Drawing for the job (mm, zero at the part's lowest x, y, z). A direction names the side the tool comes from. Give positions to 0.01 mm unless a question says otherwise; leave off trailing zeros. Write each loop counter-clockwise with the first axis right and the second up, starting at its lowest first coordinate (ties: lowest second). Pieces come first, ordered by that corner, then holes.
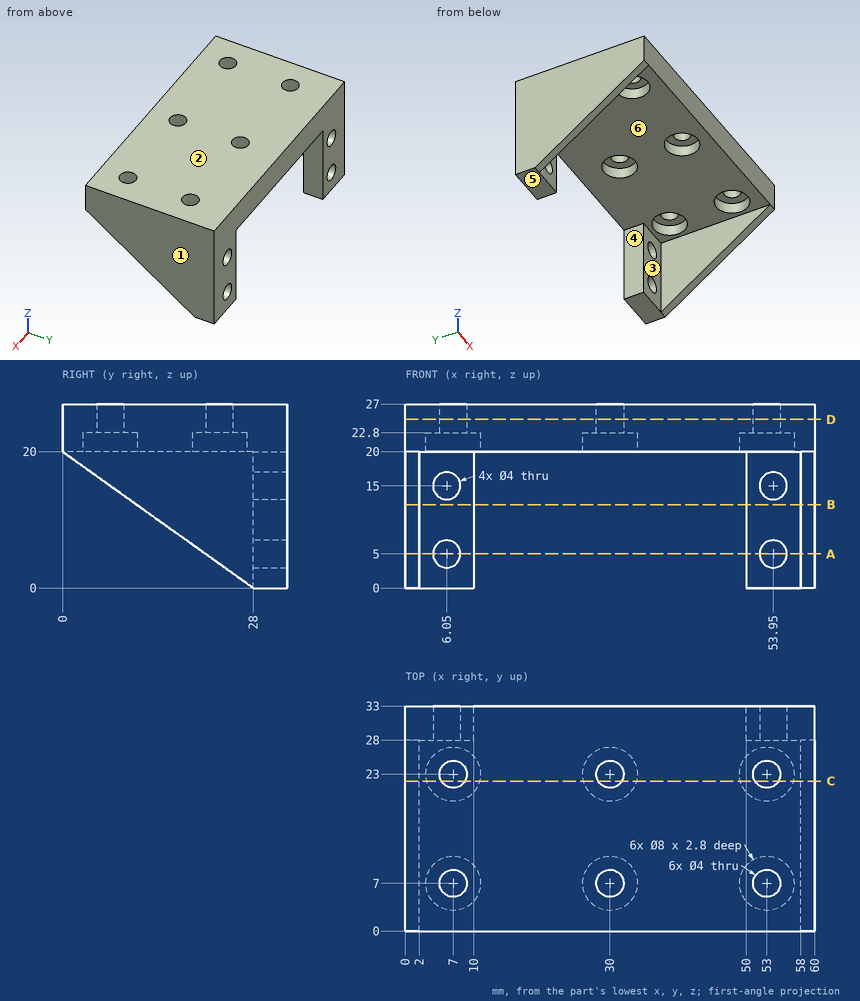
1. Which spindle directions (+Z, -Z, +X, -X, +Y, -Y) get a long thin tool onto all of the face, cutting with end or side? Do the marked faces 4, 5 and 6. Say none if no direction does.
Calculated:
face 4: -Z, +Y, -Y
face 5: -Z, +X, -X, +Y, -Y
face 6: -Z, -Y
2. Slice it at B-B, the plane z = 12.25. Write the cut outline in (x, y).
Calculated:
outline: (0, 10.85) - (2, 10.85) - (2, 28) - (10, 28) - (10, 33) - (0, 33) - close; (50, 28) - (58, 28) - (58, 10.85) - (60, 10.85) - (60, 33) - (50, 33) - close
3. Probe probe 1 along X at (y, z) = (29.35, 15); probe 2 along Y at (x, z) = (30, 21.05); probe 3 along X at (y, z) = (13.5, 13.25). List the from-to ranges inside material, lowest first.
Calculated:
probe 1: x = 0 to 4.05, 8.05 to 10, 50 to 51.95, 55.95 to 60
probe 2: y = 0 to 3, 11 to 19, 27 to 33
probe 3: x = 0 to 2, 58 to 60
4. Slice it at D-D, the plane z = 24.75. Write the cut outline in (x, y).
Calculated:
outline: (0, 0) - (60, 0) - (60, 33) - (0, 33) - close; hole circle Ø4 at (7, 7); hole circle Ø4 at (7, 23); hole circle Ø4 at (30, 7); hole circle Ø4 at (30, 23); hole circle Ø4 at (53, 7); hole circle Ø4 at (53, 23)
5. Pin check, flat tips, straight feed: P1, Ø2.5, axis at x = 54.5, y = 21.5, coming from the -Z side; P2, Ø9, axis at x = 28.5, y = 23.5, coming from the -Z side; P3, Ø5, axis at x = 53.95, z = 15, coming from the -Y side; P4, Ø2.5, axis at x = 30, y = 7, coming from the +Z side. Stop position of each tip, or through.
Calculated:
P1: stops at z = 22.8
P2: stops at z = 20
P3: stops at y = 28
P4: passes through
6. Slice it at A-A, the plane z = 5. Write the cut outline in (x, y), and give its area (3 significant figures).
Calculated:
outline: (0, 21) - (2, 21) - (2, 28) - (4.05, 28) - (4.05, 33) - (0, 33) - close; (8.05, 28) - (10, 28) - (10, 33) - (8.05, 33) - close; (50, 28) - (51.95, 28) - (51.95, 33) - (50, 33) - close; (55.95, 28) - (58, 28) - (58, 21) - (60, 21) - (60, 33) - (55.95, 33) - close
area: 88.0 mm2
7. Slice it at C-C, the plane y = 22. State how many separate pieces and enclosed holes the cut face has, and give its area (3 significant figures).
Calculated:
separate pieces: 4
enclosed holes: 0
area: 374 mm2
8. Pull direction X, two halves, no side cores. Call the marked faces 1, 2 and 3: +X half, -X half, draft (parallel to the pull), parting line (faces both ways), or undercut.
Calculated:
face 1: +X half
face 2: draft
face 3: undercut
